Autodesk Inventor part; units mm, degrees
ref_plane "YZ Plane" through (0, 0, 0) normal (1, 0, 0) x (0, 1, 0)
ref_plane "XZ Plane" through (0, 0, 0) normal (0, 1, 0) x (-1, 0, 0)
ref_plane "XY Plane" through (0, 0, 0) normal (0, 0, 1) x (1, 0, 0)
sketch "Sketch1" plane through (0, 0, 0) normal (0, 0, 1) x (1, 0, 0)
  circle A0 centre (0, 0) radius 100.508
  dimension "OuterVesselInnerdiameter" = 201.016
extrude "Extrusion1" add sketch "Sketch1" along normal blind 42
shell "Shell2" thickness 1 removed faces 0
sketch "Sketch2" plane through (0, 0, 42) normal (0, 0, 1) x (1, 0, 0)
  line L0 (0, 0) -> (-12.25, 0)
  line L1 (0, 0) -> (12.25, 0)
  point P0 (35.414, 0)
  point P1 (-35.414, 0)
  dimension "d30" = 24.5
hole "Hole1" at (-12.25, 0, 42) at (0, 0, 42) at (12.25, 0, 42) direction (0, 0, -1) diameter 5 depth 1
hole "Hole2" at (35.414, 0, 42) at (-35.414, 0, 42) direction (0, 0, -1) diameter 7 depth 1
equation "\"OuterVesselInnerdiameter\" = 4 * CrucibleThickness + 4 * CrucibleInnerDiameter"
equation "\"height\" = 1.4 * SupportHeight + 1.4 * crucible_height"
equation "\"d30\" = DistanceBetweenHolesSweep"
equation "\"d14\" = PenetrationOuterDiameter"
equation "\"d23\" = PenetrationUpstreamInnerDiameter + 2 * PenetrationUpstreamThickness"
equation "\"OuterVesselTopHolesSpacing\" = DistanceBetweenHolesSweep"
equation "\"CrucibleThickness\" = 0.254"
equation "\"CrucibleDistanceBetweenTopHoles\" = 7.62"
equation "\"OuterVesselBottomHolesSpacing\" = CrucibleThickness + 0.5 * CrucibleInnerDiameter + PenetrationUpstreamDistanceFromWallToCentre"
properties part number "outer vessel"
Model file for the job. Use its own axes, mm. A direction names the side the tool comes from. Coordinates: 2 decimals unless noted, no trailing zeros. Order: outer loops, then holes, each group sorted by start corner. A loop starts at its lowest first (then second) coordinate and runs counter-clockwise, first axis right, second up. Notation, with made-up numbers: (29.5, -25.5) -> (66.5, -25.5) arc R31 cw to (66.5, 2.5) -> close; hole circle Ø3 at (-6, 88.25). An arc over 180 degrees is marked (long way). Return JSON: item names as keys, results as strings. Group by question number.
Item 1: Saw through at D-D on x = 0. Write the cut outline in (y, z), then the cut area to 3 significant figures.
Item 2: Wall check: line 1 along Z through (x, y) = (16, 87.5); line 2 along X through (y, z) = (3, 31); line 3 along Y through (x, z) = (0, 41.35). Give the ranges that are in metal, low to high. Write a range as [from, to].
Item 3: Saw through at A-A on y = 0. Write the cut outline in (x, z).
Item 4: Saw through at B-B on x = -57. Write the cut outline in (y, z).
Item 5: Saw through at C-C on y = -34.5. Write the cut outline in (x, z).
Item 6: Tool access for faces 5 (the flat face through (21, 1, 42)), 6 (the cylindrical face through (14.7, 0.5, 41.5)), 7 (the flat face through (-1, 1, 1)): list every direction of +Z, -Z, +X, -X, +Y, -Y with a clear straight run to the whole face (end or side of a thin tool).
Item 7: Pull direction Y, two halves, no side cores. Call faces 1 (the flat face through (-1, 1, 0)), 2 (the cylindrical face through (2.44, 0.54, 41.49)), 3 (the cylindrical face through (95.867, -30.19, 20.706)), 4 (the cylindrical face through (-9.8, 0.5, 41.5)): pulls with the +Y half, pulls with the -Y half, needs draft (parallel to the pull), parting line crosses it, or undercut.
Item 8: Flat gauge pins, fed straight in: P1, Ø1.5, axis at x = -32.5, z = 18.5, coming from the +Y side; P2, Ø4.5, axis at x = 12.25, y = 0, coming from the +Z side; P3, Ø10, axis at x = -66, z = 17, coming from the +Y side. Where does each tip first touch, or does it go through?
Values found:
{
 "1": {"outline": "(-100.51, 0) -> (100.51, 0) -> (100.51, 42) -> (2.5, 42) -> (2.5, 41) -> (99.51, 41) -> (99.51, 1) -> (-99.51, 1) -> (-99.51, 41) -> (-2.5, 41) -> (-2.5, 42) -> (-100.51, 42) -> close", "area": "477 mm2"},
 "2": {"line 1": "z = [0, 1], [41, 42]", "line 2": "x = [-100.46, -99.46], [99.46, 100.46]", "line 3": "y = [-100.51, -2.5], [2.5, 100.51]"},
 "3": {"outline": "(-100.51, 0) -> (100.51, 0) -> (100.51, 42) -> (38.91, 42) -> (38.91, 41) -> (99.51, 41) -> (99.51, 1) -> (-99.51, 1) -> (-99.51, 41) -> (-38.91, 41) -> (-38.91, 42) -> (-100.51, 42) -> close; (-31.91, 41) -> (-14.75, 41) -> (-14.75, 42) -> (-31.91, 42) -> close; (-9.75, 41) -> (-2.5, 41) -> (-2.5, 42) -> (-9.75, 42) -> close; (2.5, 41) -> (9.75, 41) -> (9.75, 42) -> (2.5, 42) -> close; (14.75, 41) -> (31.91, 41) -> (31.91, 42) -> (14.75, 42) -> close"},
 "4": {"outline": "(-82.78, 0) -> (82.78, 0) -> (82.78, 42) -> (-82.78, 42) -> close; hole (-81.56, 1) -> (81.56, 1) -> (81.56, 41) -> (-81.56, 41) -> close"},
 "5": {"outline": "(-94.4, 0) -> (94.4, 0) -> (94.4, 42) -> (-94.4, 42) -> close; hole (-93.34, 1) -> (93.34, 1) -> (93.34, 41) -> (-93.34, 41) -> close"},
 "6": {"face 5": "+Z, +X, -X, +Y, -Y", "face 6": "+Z", "face 7": "none"},
 "7": {"face 1": "needs draft", "face 2": "undercut", "face 3": "parting line crosses it", "face 4": "undercut"},
 "8": {"P1": "stops at y = 95.36", "P2": "stops at z = 1", "P3": "stops at y = 79.88"}
}
